from build123d import *

# Parameters (mm, degrees)
ESQUISSE2_R        = 2.5
ESQUISSE2_R_2      = 7.5
ESQUISSE2_R_3      = 1.5
BOSS_EXTRU_5_DEPTH = 5


with BuildPart() as part:
    # Esquisse2 → Boss.-Extru.5 (new body)
    with BuildSketch(Plane(origin=(0, 0, 0), x_dir=(1, 0, 0), z_dir=(0, 1, 0))):
        with BuildLine():
            Line((-75.214465703, -26.391441925), (-75.214465703, -31.391441925))
            Line((-75.214465703, -31.391441925), (-15.214465703, -31.391441925))
            Line((-15.214465703, -31.391441925), (-15.214465703, -26.391441925))
            Line((-15.214465703, -26.391441925), (24.785534297, -26.391441925))
            Line((24.785534297, -26.391441925), (24.785534297, -31.391441925))
            Line((24.785534297, -31.391441925), (51.321432682, -31.391441925))
            ThreePointArc((51.321432682, -31.391441925), (54.785534297, -33.391441925), (58.249635912, -31.391441925))
            Line((58.249635912, -31.391441925), (84.785534297, -31.391441925))
            Line((84.785534297, -31.391441925), (84.785534297, -26.391441925))
            Line((84.785534297, -26.391441925), (119.785534297, -26.391441925))
            Line((119.785534297, -26.391441925), (119.785534297, -8.891441925))
            Line((119.785534297, -8.891441925), (124.785534297, -8.891441925))
            Line((124.785534297, -8.891441925), (124.785534297, 11.108558075))
            Line((124.785534297, 11.108558075), (119.785534297, 11.108558075))
            Line((119.785534297, 11.108558075), (119.785534297, 28.608558075))
            Line((119.785534297, 28.608558075), (-110.214465703, 28.608558075))
            Line((-110.214465703, 28.608558075), (-110.214465703, 11.108558075))
            Line((-110.214465703, 11.108558075), (-115.214465703, 11.108558075))
            Line((-115.214465703, 11.108558075), (-115.214465703, -8.891441925))
            Line((-115.214465703, -8.891441925), (-110.214465703, -8.891441925))
            Line((-110.214465703, -8.891441925), (-110.214465703, -26.391441925))
            Line((-110.214465703, -26.391441925), (-75.214465703, -26.391441925))
        make_face()
        with Locations(Location((54.785534297, -29.391441925, 0), (0, 0, 270))):
            Circle(ESQUISSE2_R, mode=Mode.SUBTRACT)
        with Locations(Location((-90.214465703, -3.891441925, 0), (0, 0, 270))):
            Circle(ESQUISSE2_R_2, mode=Mode.SUBTRACT)
        with Locations(Location((99.785534297, -3.891441925, 0), (0, 0, 270))):
            Circle(ESQUISSE2_R_2, mode=Mode.SUBTRACT)
        with Locations(Location((-105.214465703, 3.608558075, 0), (0, 0, 270))):
            Circle(ESQUISSE2_R_3, mode=Mode.SUBTRACT)
        with Locations(Location((-75.214465703, 3.608558075, 0), (0, 0, 270))):
            Circle(ESQUISSE2_R_3, mode=Mode.SUBTRACT)
        with Locations(Location((-96.714465703, 16.108558075, 0), (0, 0, 270))):
            Circle(ESQUISSE2_R_3, mode=Mode.SUBTRACT)
        with Locations(Location((-83.714465703, 16.108558075, 0), (0, 0, 270))):
            Circle(ESQUISSE2_R_3, mode=Mode.SUBTRACT)
        with Locations(Location((84.785534297, 3.608558075, 0), (0, 0, 270))):
            Circle(ESQUISSE2_R_3, mode=Mode.SUBTRACT)
        with Locations(Location((114.785534297, 3.608558075, 0), (0, 0, 270))):
            Circle(ESQUISSE2_R_3, mode=Mode.SUBTRACT)
        with Locations(Location((93.285534297, 16.108558075, 0), (0, 0, 270))):
            Circle(ESQUISSE2_R_3, mode=Mode.SUBTRACT)
        with Locations(Location((106.285534297, 16.108558075, 0), (0, 0, 270))):
            Circle(ESQUISSE2_R_3, mode=Mode.SUBTRACT)
    extrude(amount=BOSS_EXTRU_5_DEPTH)


solid = part.part
Work out the finished part from the listing and answer in its coordinate system (mm). A direction names the side the tool comes from. Round coordinates to 2 decimals unless told otherwise and drop trailing zeros. Loops run counter-clockwise (first coordinate to the right, second up) from the corner with the lowest first, then second, coordinate; pieces in that order, holes last. Notation, with made-up numbers: (11, 46) - (17, 46) arc R11 cw to (17, 55) - close; hole circle Ø9 at (54.5, 22.25). An arc over 180 degrees is marked (long way). Use one line per item in the form item = value. Start each with the question number.
(1) Which of the six approach directions +Z, -Z, +X, -X, +Y, -Y give full straight-line access (tool end or side, diameter ignored) to faces 1 (the face through (38, 2, 31.391)), 2 (the face through (24.786, 2, 29)), 3 (the face through (-113, 2, -11.109)), 4 (the face through (71, 2, 31.391))?
(2) Find section D-D on z = 19. Determine the outline of the cut face in (x, y).
(3) Flat-ended cylindrical pins translate along their axes: P1, Ø1, axis at x = 2, y = 3.5, coming from the +Z side; P2, Ø12, axis at x = 99.79, z = 3.89, coming from the +Y side; P3, Ø2, axis at x = -51, y = 4.5, coming from the +Z side; P4, Ø1.5, axis at y = 2.5, z = 18.5, coming from the -X side. Find the tip coordinate at first contact, or state that the pin passes through.
(4) Consider line 1 (Z direction, x = -84, y = 3.55); line 2 (X direction, y = 0.7, z = 30); line 3 (X direction, y = 4.75, z = 28.5). Determine where each line is inside the solid, lowest interval first.
(5) Find section C-C on x = 0. Determine the outline of the cut face in (y, z), and give its area (3 significant figures).
(6) Find section B-B on y = 1.5. Give the number of separate pieces and of enclosed holes in the cut face, and give its area (3 significant figures).
(7) Find section A-A on z = 1.5. Determine the outline of the cut face in (x, y), and give its area (3 significant figures).
(8) Determine the mould class of faces 5 (the face through (6, 2, -28.609)), 6 (the face through (-15.214, 2, 29)), 7 (the face through (119.786, 2, 18)) for opening direction X: +X half, -X half, draft (parallel to the pull), parting line (faces both ways), or undercut.
Answer list:
q1.face_1 = +Z, -X, +Y, -Y
q1.face_2 = +Z, +Y, -Y
q1.face_3 = -Z, -X, +Y, -Y
q1.face_4 = +Z, +X, +Y, -Y
q2.outline = (-110.21, 0) - (119.79, 0) - (119.79, 5) - (-110.21, 5) - close
q3.P1 = 26.39
q3.P2 = through
q3.P3 = 31.39
q3.P4 = -110.21
q4.line_1 = -28.61 to -17.58, -14.64 to -0.31, 8.09 to 26.39
q4.line_2 = -75.21 to -15.21, 24.79 to 52.36, 57.21 to 84.79
q4.line_3 = -75.21 to -15.21, 24.79 to 52.45, 57.12 to 84.79
q5.outline = (0, -28.61) - (5, -28.61) - (5, 26.39) - (0, 26.39) - close
q5.area = 275 mm^2
q6.separate_pieces = 1
q6.enclosed_holes = 11
q6.area = 13,000 mm^2
q7.outline = (-115.21, 0) - (-97.32, 0) - (-97.32, 5) - (-115.21, 5) - close; (-83.11, 0) - (92.68, 0) - (92.68, 5) - (-83.11, 5) - close; (106.89, 0) - (124.79, 0) - (124.79, 5) - (106.89, 5) - close
q7.area = 1,060 mm^2
q8.face_5 = draft
q8.face_6 = undercut
q8.face_7 = +X half
